Read the model definition and answer for the solid it produces. Units are mm, in the model's axes. Face numbers are marked on the shaded views. Coordinates: 2 decimals unless noted, no trailing zeros. Order: outer loops, then holes, each group sorted by start corner. A loop starts at its lowest first (then second) coordinate and runs counter-clockwise, first axis right, second up. Notation, with made-up numbers: (24, -38) -> (33, -38) arc R16 ccw to (33, -19) -> close; hole circle Ø7 at (-1.5, 10.5). An arc over 180 degrees is marked (long way). Answer in a Markdown table with one row per item.
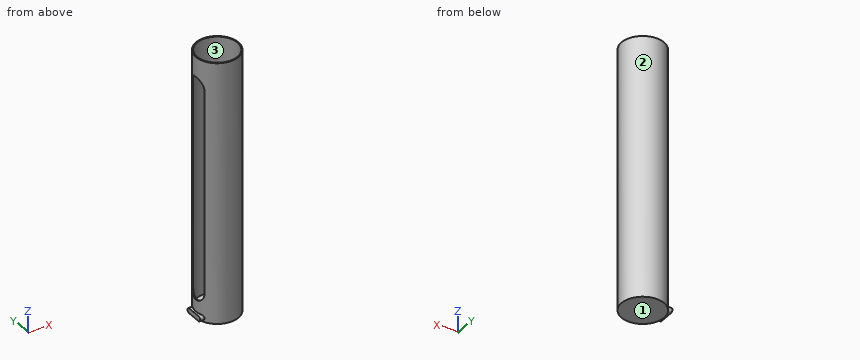
from build123d import *

# Parameters (mm, degrees)
SKETCH2_R           = 10.3759
BOSS_EXTRUDE1_DEPTH = 127
SKETCH3_R           = 9.906
CUT_EXTRUDE1_DEPTH  = 124.46
CUT_EXTRUDE2_DEPTH  = 12.7
BOSS_EXTRUDE2_DEPTH = 11.43


with BuildPart() as part:
    # Sketch2 → Boss-Extrude1 (new body)
    with BuildSketch(Plane.XY):
        Circle(SKETCH2_R)
    extrude(amount=BOSS_EXTRUDE1_DEPTH)

    # Sketch3 → Cut-Extrude1 (cut)
    with BuildSketch(Plane.XY.offset(127)):
        Circle(SKETCH3_R)
    extrude(amount=-CUT_EXTRUDE1_DEPTH, mode=Mode.SUBTRACT)

    # Sketch4 → Cut-Extrude2 (cut)
    with BuildSketch(Plane(origin=(0, 0, 0), x_dir=(0, 0, -1), z_dir=(1, 0, 0))):
        with BuildLine():
            Line((-112.627725765, 4.69603261), (-13.529396587, 4.69603261))
            ThreePointArc((-13.529396587, 4.69603261), (-8.833363977, 0), (-13.529396587, -4.69603261))
            Line((-13.529396587, -4.69603261), (-112.627725765, -4.69603261))
            ThreePointArc((-112.627725765, -4.69603261), (-117.323758375, 0), (-112.627725765, 4.69603261))
        make_face()
    extrude(amount=-CUT_EXTRUDE2_DEPTH, mode=Mode.SUBTRACT)

    # Sketch5 → Boss-Extrude2 (add)
    with BuildSketch(Plane(origin=(0, 0, 0), x_dir=(0, 0, -1), z_dir=(1, 0, 0))):
        with BuildLine():
            Line((-0.645409683, 3.552127231), (-0.645409683, -3.552127231))
            ThreePointArc((-0.645409683, -3.552127231), (-1.849520609, -4.756238156), (-3.053631534, -3.552127231))
            Line((-3.053631534, -3.552127231), (-3.053631534, 3.552127231))
            ThreePointArc((-3.053631534, 3.552127231), (-1.849520609, 4.756238156), (-0.645409683, 3.552127231))
        make_face()
    extrude(amount=-BOSS_EXTRUDE2_DEPTH)


solid = part.part
Q1. The part is cut by section C-C (x = -7). Write down the section's boundary in (y, z), then the cut area to 3 significant figures.
Outcome:
| item | result |
|---|---|
| outline | (-7.66, 0) -> (7.66, 0) -> (7.66, 127) -> (7.01, 127) -> (7.01, 2.54) -> (4.54, 2.54) arc R1.2 ccw to (3.55, 3.05) -> (-3.55, 3.05) arc R1.2 ccw to (-4.54, 2.54) -> (-7.01, 2.54) -> (-7.01, 127) -> (-7.66, 127) -> close |
| area | 205 mm² |
Q2. The part is cut by section B-B (z = 73). Write down the section's boundary in (x, y).
Outcome:
| item | result |
|---|---|
| outline | (-9.25, -4.7) arc R10.38 ccw (long way) to (-9.25, 4.7) -> (-8.72, 4.7) arc R9.91 cw (long way) to (-8.72, -4.7) -> close |
Q3. Given pin 1 (5 mm diameter, centred on x = -6.5, z = 15.5, fed in from -Y); pin 2 (6 mm diameter, centred on y = 5, z = 88, fed in from +X); pin 3 (2 mm diameter, centred on x = -2.5, y = 0, fed in from +Z), each flat-ended and moving along its own axis, determine where each tip first touches the part or whether it passes through.
Outcome:
| item | result |
|---|---|
| pin 1 | y = -9.57 |
| pin 2 | x = 10.18 |
| pin 3 | z = 3.05 |
Q4. The part is cut by section A-A (y = 0). Write down the section's boundary in (x, z), then the cut area to 3 significant figures.
Outcome:
| item | result |
|---|---|
| outline | (-11.43, 0.65) -> (-10.38, 0.65) -> (-10.38, 0) -> (10.38, 0) -> (10.38, 127) -> (9.91, 127) -> (9.91, 2.54) -> (0, 2.54) -> (0, 3.05) -> (-9.91, 3.05) -> (-9.91, 8.83) -> (-10.38, 8.83) -> (-10.38, 3.05) -> (-11.43, 3.05) -> close; (-10.38, 117.32) -> (-9.91, 117.32) -> (-9.91, 127) -> (-10.38, 127) -> close |
| area | 126 mm² |
Q5. For a pull along X with two mould halves and no side action, classify the marked faces 1, 2 and 3 as pulls with the +X half, pulls with the -X half, needs draft (parallel to the pull), parting line crosses it, or undercut.
Outcome:
| item | result |
|---|---|
| face 1 | needs draft |
| face 2 | parting line crosses it |
| face 3 | undercut |
Q6. The part is cut by section D-D (y = 7.5). Write down the section's boundary in (x, z).
Outcome:
| item | result |
|---|---|
| outline | (-7.17, 0) -> (7.17, 0) -> (7.17, 127) -> (6.47, 127) -> (6.47, 2.54) -> (-6.47, 2.54) -> (-6.47, 127) -> (-7.17, 127) -> close |
Q7. Consider line 1 (Y direction, x = 0, z = 64); line 2 (Z direction, x = 5, y = 5.25); line 3 (Y direction, x = 4.25, z = 116.5). Determine where each line is inside the solid, lowest interval first.
Outcome:
| item | result |
|---|---|
| line 1 | -10.38 to -9.91, 9.91 to 10.38 |
| line 2 | 0 to 2.54 |
| line 3 | -9.47 to -8.95, 8.95 to 9.47 |
